```python
from build123d import *

# Parameters (mm, degrees)
F1_DEPTH = 9.3
F0_R     = 6
F2_DEPTH = 4.3
F0_R_2   = 2.3
F3_DEPTH = 2.8
F5_DEPTH = 5.26
F6_DEPTH = 5.26
F8_DEPTH = 5.26
F9_DEPTH = 5.26


with BuildPart() as f1:
    # F0 (on Top) → F1 (new body)
    with BuildSketch(Plane.XY):
        Polygon((36.2151488662, -0.8635242283), (33.6151488662, -0.8635242283), (33.6151488662, -6.1235242283), (30.6651488662, -6.1235242283), (30.6651488662, -13.1035242283), (33.6151488662, -13.1035242283), (33.6151488662, -18.3635242283), (36.2151488662, -18.3635242283), align=None)
    extrude(amount=F1_DEPTH)



with BuildPart() as f1b:
    # F0 (on Top) → F1, piece 2 (new body)
    with BuildSketch(Plane.XY):
        Polygon((14.0851488662, -0.8635242283), (11.4851488662, -0.8635242283), (11.4851488662, -18.3635242283), (14.0851488662, -18.3635242283), (14.0851488662, -13.1035242283), (17.0351488662, -13.1035242283), (17.0351488662, -6.1235242283), (14.0851488662, -6.1235242283), align=None)
    extrude(amount=F1_DEPTH)


with BuildPart() as f1_1:
    add(f1.part)

    add(f1b.part)  # F2 merges F1b
    # F0 (on Top) → F2 (join)
    with BuildSketch(Plane.XY):
        Polygon((30.6651488662, -0.8635242283), (17.0351488662, -0.8635242283), (17.0351488662, -6.1235242283), (17.0351488662, -13.1035242283), (17.0351488662, -18.3635242283), (30.6651488662, -18.3635242283), (30.6651488662, -13.1035242283), (30.6651488662, -6.1235242283), align=None)
        with Locations((23.8501488662, -9.6135242283)):
            Circle(F0_R, mode=Mode.SUBTRACT)
    extrude(amount=F2_DEPTH)

    # F0 (on Top) → F3 (join)
    with BuildSketch(Plane.XY):
        with Locations((23.8501488662, -9.6135242283)):
            Circle(F0_R)
        with Locations((23.8501488662, -9.6135242283)):
            Circle(F0_R_2, mode=Mode.SUBTRACT)
    extrude(amount=F3_DEPTH)

    # F4 (on face) → F5 (join)
    with BuildSketch(Plane.XZ.offset(13.1035242283)):
        Polygon((15.3120337054, 7.5), (17.0351488662, 7.5), (17.0351488662, 9.3), (14.0851488662, 9.3), (14.0851488662, 7.5), align=None)
    extrude(amount=F5_DEPTH)

    # F4 (on face) → F6 (join)
    with BuildSketch(Plane.XZ.offset(13.1035242283)):
        Polygon((32.3882640269, 7.5), (33.6151488662, 7.5), (33.6151488662, 9.3), (30.6651488662, 9.3), (30.6651488662, 7.5), align=None)
    extrude(amount=F6_DEPTH)

    # F7 (on face) → F8 (join)
    with BuildSketch(Plane(origin=(0, -6.1235242283, 0), x_dir=(-1, 0, 0), z_dir=(0, 1, 0))):
        Polygon((-32.1401488662, 7.5), (-30.6651488662, 7.5), (-30.6651488662, 9.3), (-33.6151488662, 9.3), (-33.6151488662, 7.5), align=None)
    extrude(amount=F8_DEPTH)

    # F7 (on face) → F9 (join)
    with BuildSketch(Plane(origin=(0, -6.1235242283, 0), x_dir=(-1, 0, 0), z_dir=(0, 1, 0))):
        Polygon((-15.5601488662, 7.5), (-14.0851488662, 7.5), (-14.0851488662, 9.3), (-17.0351488662, 9.3), (-17.0351488662, 7.5), align=None)
    extrude(amount=F9_DEPTH)


solid = f1_1.part
```
Geometry: final body of the model. Coordinates: model frame, mm. A direction names the side the tool comes from. Round coordinates to 2 decimals unless told otherwise and drop trailing zeros. Order: outer loops, then holes, each group sorted by start corner. A loop starts at its lowest first (then second) coordinate and runs counter-clockwise, first axis right, second up. Notation, with made-up numbers: (59, 26) -> (116, 26) arc R15 cw to (116, 51) -> close; hole circle Ø7 at (47, 68.25). An arc over 180 degrees is marked (long way). Use one line per item in the form item = value.
(1) Section A-A on z = 6.25. Return loops of the section in (x, y).
Results list:
outline = (11.49, -18.36) -> (14.09, -18.36) -> (14.09, -13.1) -> (17.04, -13.1) -> (17.04, -6.12) -> (14.09, -6.12) -> (14.09, -0.86) -> (11.49, -0.86) -> close; (30.67, -13.1) -> (33.62, -13.1) -> (33.62, -18.36) -> (36.22, -18.36) -> (36.22, -0.86) -> (33.62, -0.86) -> (33.62, -6.12) -> (30.67, -6.12) -> close
(2) Draft query along X for faces 1 (the face through (17.035, -3, 2)), 2 (the face through (11.485, -9, 5)), 3 (the face through (33, -10, 9.3)). Return one class per face: pulls with the +X half, pulls with the -X half, needs draft (parallel to the pull), parting line crosses it, or undercut.
Results list:
face_1 = undercut
face_2 = pulls with the -X half
face_3 = needs draft
(3) Section C-C on y = -4.75. Return loops of the section in (x, z), and give its area (3 significant figures).
Results list:
outline = (11.49, 0) -> (14.09, 0) -> (14.09, 7.5) -> (17.04, 7.5) -> (17.04, 9.3) -> (11.49, 9.3) -> close; (17.04, 0) -> (30.67, 0) -> (30.67, 4.3) -> (27.36, 4.3) -> (27.36, 2.8) -> (20.34, 2.8) -> (20.34, 4.3) -> (17.04, 4.3) -> close; (30.67, 7.5) -> (33.62, 7.5) -> (33.62, 0) -> (36.22, 0) -> (36.22, 9.3) -> (30.67, 9.3) -> close
area = 107 mm^2
(4) First-contact query: pin 1 Ø2.5 at (x, z) = (32, 5) entering from +Y; pin 2 Ø2.5 at (x, z) = (15.5, 5) entering from -Y; pin 3 Ø6 at (x, y) = (21, -8) entering from +Z. Flat tips, straight axial feed; report the tip coordinate or a pass-through.
Results list:
pin_1 = -6.12
pin_2 = -13.1
pin_3 = 4.3
(5) Ray query, probe 1 along X at (y, z) = (-11.75, 6.75); probe 2 along X at (y, z) = (-2.25, 2.75); probe 3 along X at (y, z) = (-17.5, 6). Return the intervals inside material, ascending. Write a range as [from, to].
Results list:
probe_1 = [11.49, 17.04], [30.67, 36.22]
probe_2 = [11.49, 14.09], [17.04, 30.67], [33.62, 36.22]
probe_3 = [11.49, 14.09], [33.62, 36.22]
(6) Section D-D on z = 0.5. Return loops of the section in (x, y), and give its area (3 significant figures).
Results list:
outline = (11.49, -18.36) -> (14.09, -18.36) -> (14.09, -13.1) -> (17.04, -13.1) -> (17.04, -18.36) -> (30.67, -18.36) -> (30.67, -13.1) -> (33.62, -13.1) -> (33.62, -18.36) -> (36.22, -18.36) -> (36.22, -0.86) -> (33.62, -0.86) -> (33.62, -6.12) -> (30.67, -6.12) -> (30.67, -0.86) -> (17.04, -0.86) -> (17.04, -6.12) -> (14.09, -6.12) -> (14.09, -0.86) -> (11.49, -0.86) -> close; hole circle Ø4.6 at (23.85, -9.61)
area = 354 mm^2
(7) Access query for faces 4 (the face through (26.4, -9.5, 2.8)), 5 (the face through (30.665, -10, 7)), 6 (the face through (16, -4, 7.5)), 7 (the face through (17.035, -16, 2)). Directions: +Z, -Z, +X, -X, +Y, -Y. A direction counts if a zero-diameter tool reaches every point of the face in a straight line with its end or side. Return the directions, or none.
Results list:
face_4 = +Z
face_5 = +Z, +Y, -Y
face_6 = -Z, +Y
face_7 = -Z, -Y
(8) Section B-B on x = 15.5. Return loops of the section in (y, z).
Results list:
outline = (-18.36, 7.5) -> (-13.1, 7.5) -> (-13.1, 0) -> (-6.12, 0) -> (-6.12, 7.5) -> (-0.86, 7.5) -> (-0.86, 9.3) -> (-18.36, 9.3) -> close
